from build123d import *

# Parameters (mm, degrees)
F0_W     = 1524
F0_H     = 2032
F1_DEPTH = 609.6
F2_R     = 50.8
F3_W     = 1600.2
F3_H     = 2184.4
F4_DEPTH = 304.8


with BuildPart() as f1:
    # F0 (on Top) → F1 (new body)
    with BuildSketch(Plane.XY):
        with Locations((-762, 1016)):
            Rectangle(F0_W, F0_H)
    extrude(amount=F1_DEPTH)

    # F2
    f2_edges = [f1.edges().sort_by_distance(p)[0] for p in [
        (-762, 0, 609.6),
        (-1524, 1016, 609.6),
        (0, 1016, 609.6),
    ]]
    fillet(f2_edges, radius=F2_R)

    # F3 (on Top) → F4 (join)
    with BuildSketch(Plane.XY):
        with Locations((-762, 1016)):
            Rectangle(F3_W, F3_H)
    extrude(amount=F4_DEPTH)


solid = f1.part
Input: part model. Units: mm. Frame: model coordinates. A direction names the side the tool comes from. Coordinates: 2 decimals unless noted, no trailing zeros. Order: outer loops, then holes, each group sorted by start corner. A loop starts at its lowest first (then second) coordinate and runs counter-clockwise, first axis right, second up.
1. Cut plane C-C, the plane z = 521. Return loops of the section in (x, y).
Checked values:
outline: (-1524, 0) - (0, 0) - (0, 2032) - (-1524, 2032) - close
2. Cut plane B-B, the plane y = 1955. Return loops of the section in (x, z).
Checked values:
outline: (-1562.1, 0) - (38.1, 0) - (38.1, 304.8) - (0, 304.8) - (0, 558.8) arc R50.8 ccw to (-50.8, 609.6) - (-1473.2, 609.6) arc R50.8 ccw to (-1524, 558.8) - (-1524, 304.8) - (-1562.1, 304.8) - close
3. Contact query for flat-ended pins moving along their axis: P1, Ø1, axis at x = -718.5, z = 509, coming from the -Y side; P2, Ø10, axis at x = -1297, y = 372.5, coming from the -Z side. Output: stop coordinate, or through.
Checked values:
P1: stops at y = 0
P2: stops at z = 0
4. Access query for faces 1 (the flat face through (-773, 0, 430)), 2 (the flat face through (-773, 2032, 455)), 3 (the flat face through (-1524, 1002, 430)), 4 (the flat face through (0, 1002, 430)). Directions: +Z, -Z, +X, -X, +Y, -Y. A direction counts if a zero-diameter tool reaches every point of the face in a straight line with its end or side. Return the directions, or none.
Checked values:
face 1: +Z, +X, -X, -Y
face 2: +Z, +X, -X, +Y
face 3: +Z, -X, +Y, -Y
face 4: +Z, +X, +Y, -Y
5. Cut plane A-A, the plane x = -120.5. Return loops of the section in (y, z).
Checked values:
outline: (-76.2, 0) - (2108.2, 0) - (2108.2, 304.8) - (2032, 304.8) - (2032, 609.6) - (50.8, 609.6) arc R50.8 ccw to (0, 558.8) - (0, 304.8) - (-76.2, 304.8) - close
6. Ray query, line 1 along X through (y, z) = (1132, 325.5); line 2 along Y through (x, z) = (-1255, 513); line 3 along X through (y, z) = (385.5, 565.5). Return the intervals inside material, ascending.
Checked values:
line 1: x = -1524 to 0
line 2: y = 0 to 2032
line 3: x = -1523.56 to -0.44
